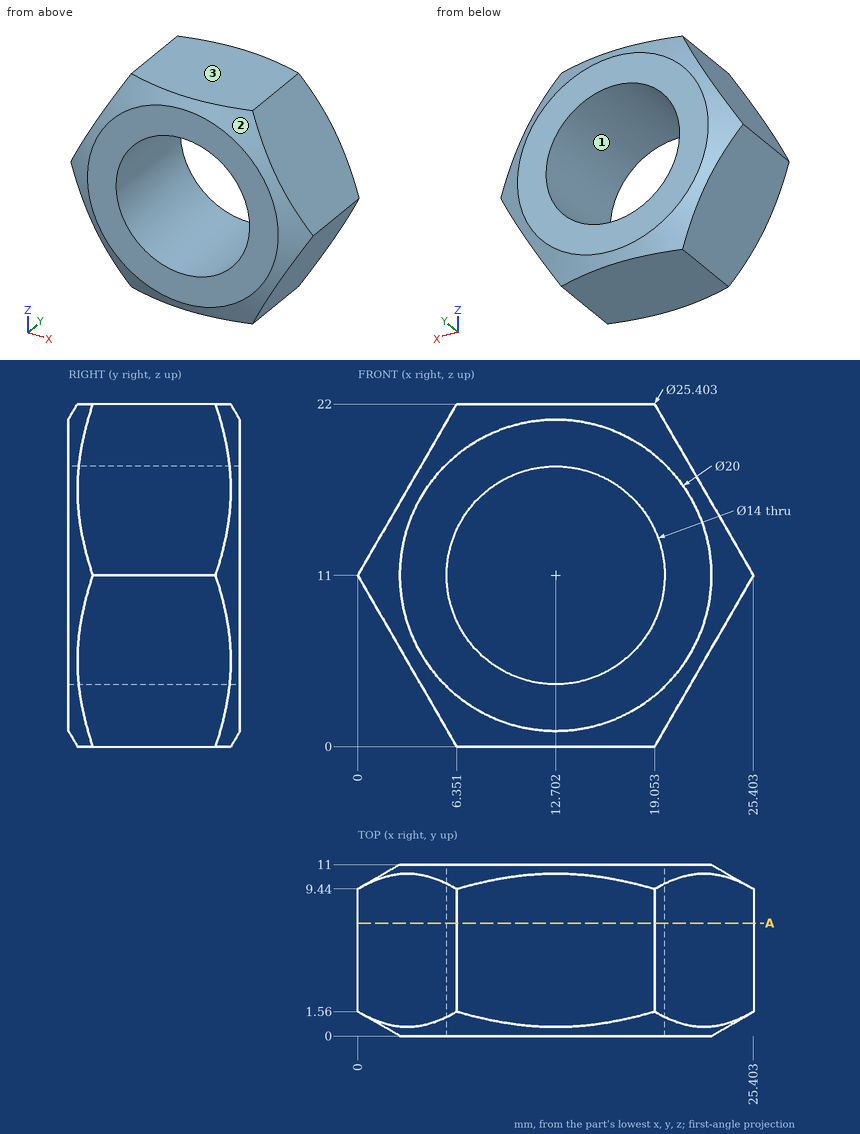
Verification items for this drawing (mm, ordinates from the low corner). Give positions to 0.01 mm unless a question says otherwise; leave off trailing zeros. Order: outer loops, then holes, each group sorted by start corner. A loop starts at its lowest first (then second) coordinate and runs counter-clockwise, first axis right, second up. Notation, with made-up numbers: M -37.5,-30 L -19.5,-30 A19 cw -19.5,-17 Z; hole C 73.5,9 d4. An arc over 180 degrees is marked long. Use a Markdown table: item, result.
Item 1: Section check A-A (y = 7.25). Record the cut outline in (x, z), and give its area (3 significant figures).
Answers follow:
| item | result |
|---|---|
| outline | M 0,11 L 6.35,0 L 19.05,0 L 25.4,11 L 19.05,22 L 6.35,22 Z; hole C 12.7,11 d14 |
| area | 265 mm2 |
Item 2: Depth check by flat-ended pin: P1, Ø1.5, axis at x = 3, y = 5, coming from the +Z side (1 decimal); P2, Ø11, axis at x = 12.7, z = 11, coming from the -Y side; P3, Ø3, axis at x = 15, y = 1.5, coming from the -Z side; P4, Ø1.5, axis at y = 7.5, z = 16.5, coming from the +X side. Enter the tip coordinate at first touch or a pass-through.
Answers follow:
| item | result |
|---|---|
| P1 | stops at z = 17.5 |
| P2 | passes through |
| P3 | stops at z = 0 |
| P4 | stops at x = 22.66 |
Item 3: Draft check along Z on the marked faces 1, 2 and 3. Enter one of: +Z half, -Z half, draft (parallel to the pull), parting line (faces both ways), or undercut.
Answers follow:
| item | result |
|---|---|
| face 1 | undercut |
| face 2 | parting line |
| face 3 | +Z half |
Item 4: Material ranges on line 1 along Z through (x, y) = (14.25, 0.5) (1 decimal); line 2 along Z through (x, y) = (13, 7.5); line 3 along X through (y, z) = (3.25, 11.25) (1 decimal), recorded low to high.
Answers follow:
| item | result |
|---|---|
| line 1 | z = 0.2 to 4.2, 17.8 to 21.8 |
| line 2 | z = 0 to 4.01, 17.99 to 22 |
| line 3 | x = 0.1 to 5.7, 19.7 to 25.3 |
